```python
from build123d import *
from build123d.topology import SkipClean

# Parameters (mm, degrees)
SKETCH1_R                             = 20
FIRST_EXTRUDE_FOR_RUBBER_PIECE_DEPTH  = 1
SECOND_EXTRUDE_FOR_RUBBER_PIECE_DEPTH = 7
HOLE_FOR_SCREW_RUBBER_DEPTH           = 23
HOLE_FOR_SCREW_RUBBER_DEPTH_BACK      = 15
SKETCH3_R                             = 1


with BuildPart() as part:
    # Sketch1 → First Extrude for Rubber Piece (new body)
    with BuildSketch(Plane(origin=(0, 0, 0), x_dir=(1, 0, 0), z_dir=(0, 1, 0))):
        with Locations(Location((0, 0, 0), (0, 0, 270))):
            Circle(SKETCH1_R)
    extrude(amount=FIRST_EXTRUDE_FOR_RUBBER_PIECE_DEPTH)

    # Sketch2 → Second Extrude for Rubber Piece (add)
    with SkipClean():  # the faces are left unmerged after this step: merging them gives an invalid solid
        with BuildSketch(Plane(origin=(0, 1, 0), x_dir=(1, 0, 0), z_dir=(0, 1, 0))):
            with BuildLine():
                ThreePointArc((-2.5, 0), (-2.414814566, 0.647047613), (-2.165063509, 1.25))
                Line((-2.165063509, 1.25), (-17.320508076, 10))
                ThreePointArc((-17.320508076, 10), (-19.318516526, 5.176380902), (-20, 0))
                Line((-20, 0), (-2.5, 0))
            make_face()
            with BuildLine():
                ThreePointArc((-1.767766953, 1.767766953), (-1.25, 2.165063509), (-0.647047613, 2.414814566))
                Line((-0.647047613, 2.414814566), (-5.176380902, 19.318516526))
                ThreePointArc((-5.176380902, 19.318516526), (-10, 17.320508076), (-14.142135624, 14.142135624))
                Line((-14.142135624, 14.142135624), (-1.767766953, 1.767766953))
            make_face()
            with BuildLine():
                Line((0, 20), (0, 2.5))
                ThreePointArc((0, 2.5), (0.647047613, 2.414814566), (1.25, 2.165063509))
                Line((1.25, 2.165063509), (10, 17.320508076))
                ThreePointArc((10, 17.320508076), (5.176380902, 19.318516526), (0, 20))
            make_face()
            with BuildLine():
                Line((14.142135624, 14.142135624), (1.767766953, 1.767766953))
                ThreePointArc((1.767766953, 1.767766953), (2.165063509, 1.25), (2.414814566, 0.647047613))
                Line((2.414814566, 0.647047613), (19.318516526, 5.176380902))
                ThreePointArc((19.318516526, 5.176380902), (17.320508076, 10), (14.142135624, 14.142135624))
            make_face()
            with BuildLine():
                Line((20, 0), (2.5, 0))
                ThreePointArc((2.5, 0), (2.414814566, -0.647047613), (2.165063509, -1.25))
                Line((2.165063509, -1.25), (17.320508076, -10))
                ThreePointArc((17.320508076, -10), (19.318516526, -5.176380902), (20, 0))
            make_face()
            with BuildLine():
                Line((14.142135624, -14.142135624), (1.767766953, -1.767766953))
                ThreePointArc((1.767766953, -1.767766953), (1.25, -2.165063509), (0.647047613, -2.414814566))
                Line((0.647047613, -2.414814566), (5.176380902, -19.318516526))
                ThreePointArc((5.176380902, -19.318516526), (10, -17.320508076), (14.142135624, -14.142135624))
            make_face()
            with BuildLine():
                ThreePointArc((0, -2.5), (-0.647047613, -2.414814566), (-1.25, -2.165063509))
                Line((-1.25, -2.165063509), (-10, -17.320508076))
                ThreePointArc((-10, -17.320508076), (-5.176380902, -19.318516526), (0, -20))
                Line((0, -20), (0, -2.5))
            make_face()
            with BuildLine():
                ThreePointArc((-1.767766953, -1.767766953), (-2.165063509, -1.25), (-2.414814566, -0.647047613))
                Line((-2.414814566, -0.647047613), (-19.318516526, -5.176380902))
                ThreePointArc((-19.318516526, -5.176380902), (-17.320508076, -10), (-14.142135624, -14.142135624))
                Line((-14.142135624, -14.142135624), (-1.767766953, -1.767766953))
            make_face()
        extrude(amount=SECOND_EXTRUDE_FOR_RUBBER_PIECE_DEPTH)

    # Sketch3 → Hole for Screw _Rubber (cut, two sides: drawn at the far end of the back side and taken through both)
    with SkipClean():  # the faces are left unmerged after this step: merging them gives an invalid solid
        with BuildSketch(Plane(origin=(0, 1, 0), x_dir=(1, 0, 0), z_dir=(0, 1, 0)).offset(-HOLE_FOR_SCREW_RUBBER_DEPTH_BACK)):
            with Locations(Location((0, 0, 0), (0, 0, 270))):
                Circle(SKETCH3_R)
        extrude(amount=HOLE_FOR_SCREW_RUBBER_DEPTH + HOLE_FOR_SCREW_RUBBER_DEPTH_BACK, mode=Mode.SUBTRACT)


solid = part.part
```
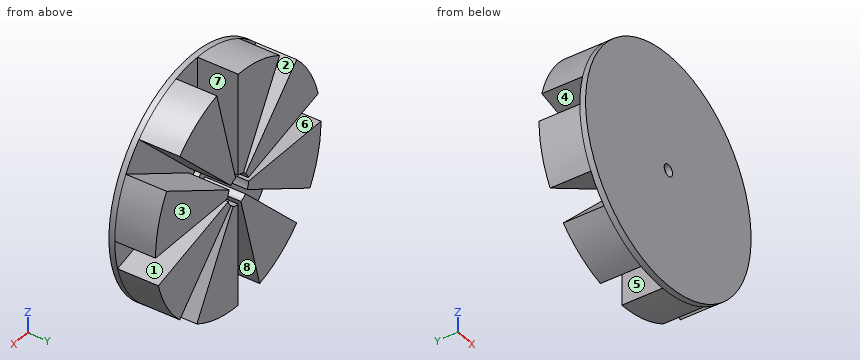
Part model, mm, in its own coordinate system. Face numbers are marked on the shaded views. A direction names the side the tool comes from. Coordinates: 2 decimals unless noted, no trailing zeros. Write each loop counter-clockwise with the first axis right and the second up, starting at its lowest first coordinate (ties: lowest second). Pieces come first, ordered by that corner, then holes.
Item 1: Slice it at B-B (z = 13). Write the cut outline in (x, y), and give its area (3 significant figures).
Item 2: Probe line 1 (Z direction, x = 12, y = 4.75); line 2 (X direction, y = 0.55, z = 0); line 3 (Z direction, x = 11.5, y = 3). List the from-to ranges inside material, lowest first.
Item 3: Slice it at D-D (x = -16). Write the cut outline in (y, z), and give its area (3 significant figures).
Item 4: Slice it at C-C (x = 7.5). Write the cut outline in (y, z).
Item 5: Mould opens along Z. For the marked faces 6, 7 and 8 say: released by +Z, released by -Z, zero draft, split by the parting line, or undercut.
Item 6: Which spindle directions (+Z, -Z, +X, -X, +Y, -Y) get a long thin tool onto all of the face, cutting with end or side? Do the marked faces 1, 2, 3, 4 and 5. Say none if no direction does.
Item 7: Pin check, flat tip, straight feed: pin 1 (1.5 mm diameter, centred on y = 5.5, z = 1.5, fed in from +X). Stop position of the tip, or through.
Item 8: Slice it at A-A (y = 2.75). Count the separate pieces of the cut face and the enclosed holes in it, and give its area (3 significant figures).
Results found:
1. outline: (-15.2, 0) - (15.2, 0) - (15.2, 1) - (13, 1) - (13, 8) - (3.48, 8) - (3.48, 1) - (0, 1) - (0, 8) - (-7.51, 8) - (-7.51, 1) - (-13, 1) - (-13, 8) - (-15.2, 8) - close
1. area: 165 mm2
2. line 1: z = -12 to -3.22, 0 to 6.93, 12 to 16
2. line 2: x = -20 to -1, 1 to 20
2. line 3: z = -11.5 to -3.08, 0 to 6.64, 11.5 to 16.36
3. outline: (0, -12) - (1, -12) - (1, -9.24) - (8, -9.24) - (8, 0) - (1, 0) - (1, 4.29) - (8, 4.29) - (8, 12) - (0, 12) - close
3. area: 143 mm2
4. outline: (0, -18.54) - (8, -18.54) - (8, -12.99) - (1, -12.99) - (1, -7.5) - (8, -7.5) - (8, -2.01) - (1, -2.01) - (1, 0) - (8, 0) - (8, 4.33) - (1, 4.33) - (1, 7.5) - (8, 7.5) - (8, 18.54) - (0, 18.54) - close
5. face 6: undercut
5. face 7: zero draft
5. face 8: released by -Z
6. face 1: +X, +Y
6. face 2: +Y
6. face 3: +Z, -Z, +X, -X, +Y
6. face 4: -X, +Y
6. face 5: -Z, +Y
7. pin 1: stops at x = 19.99
8. separate pieces: 8
8. enclosed holes: 0
8. area: 825 mm2
